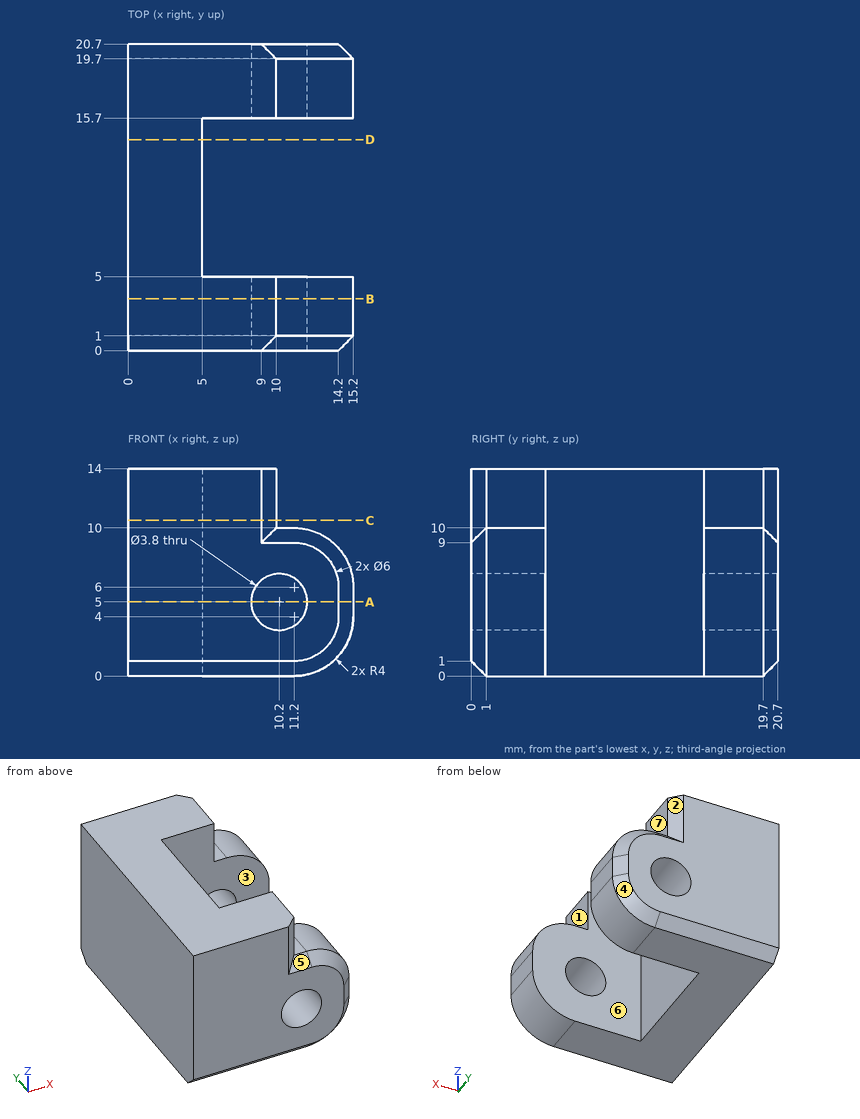
Geometry: see drawing. Coordinates: mm, zero at the bounding-box minimum. A direction names the side the tool comes from. Coordinates: 2 decimals unless noted, no trailing zeros. Loops run counter-clockwise (first coordinate to the right, second up) from the corner with the lowest first, then second, coordinate; pieces in that order, holes last. Notation, with made-up numbers: M 6.25,28 L 58.25,28 A25 cw 58.25,51 Z; hole C 57.25,5.25 d4. An arc over 180 degrees is marked long. Answer in a Markdown table with one row per item.
Q1. Draft query along Y for the marked faces 4, 5, 6 and 7. Return one class per face: pulls with the +Y half, pulls with the -Y half, needs draft (parallel to the pull), parting line crosses it, or undercut.
Answers below:
| item | result |
|---|---|
| face 4 | pulls with the +Y half |
| face 5 | pulls with the -Y half |
| face 6 | undercut |
| face 7 | needs draft |
Q2. Set-up query: the marked faces 1, 2 and 3. Return all of +Z, -Z, +X, -X, +Y, -Y with unobstructed straight access to the full face (end or side cutting, diameter ignored); none if empty.
Answers below:
| item | result |
|---|---|
| face 1 | +Z, +X, +Y, -Y |
| face 2 | +Z, +X, +Y |
| face 3 | +Z, -Z, +X |
Q3. Ray query, probe 1 along Z at (x, y) = (10.2, 3.65); probe 2 along Y at (x, z) = (6, 13); probe 3 along X at (y, z) = (14, 6.5). Return the intervals inside material, ascending. Write a range as from..to.
Answers below:
| item | result |
|---|---|
| probe 1 | z = 0..3.1, 6.9..10 |
| probe 2 | y = 0..5, 15.7..20.7 |
| probe 3 | x = 0..5 |
Q4. Section B-B on y = 3.5. Return the cut outline in (x, z), plus the area to 3 significant figures.
Answers below:
| item | result |
|---|---|
| outline | M 0,0 L 11.2,0 A4 ccw 15.2,4 L 15.2,6 A4 ccw 11.2,10 L 10,10 L 10,14 L 0,14 Z; hole C 10.2,5 d3.8 |
| area | 174 mm^2 |
Q5. Section A-A on z = 5. Return the cut outline in (x, y).
Answers below:
| item | result |
|---|---|
| outline | M 0,0 L 8.3,0 L 8.3,5 L 5,5 L 5,15.7 L 8.3,15.7 L 8.3,20.7 L 0,20.7 Z; M 12.1,0 L 14.2,0 L 15.2,1 L 15.2,5 L 12.1,5 Z; M 12.1,15.7 L 15.2,15.7 L 15.2,19.7 L 14.2,20.7 L 12.1,20.7 Z |
Q6. First-contact query: pin 1 (3 mm diameter, centred on x = 9.5, z = 9.5, fed in from -Y); pin 2 (5 mm diameter, centred on x = 12, y = 13.5, fed in from +Z); pin 3 (1.2 mm diameter, centred on y = 18.5, z = 12, fed in from +X); pin 4 (5 mm diameter, centred on x = 8, y = 12, fed in from +Z). Flat tips, straight axial feed; report the tip coordinate or a pass-through.
Answers below:
| item | result |
|---|---|
| pin 1 | stops at y = 0 |
| pin 2 | stops at z = 10 |
| pin 3 | stops at x = 10 |
| pin 4 | passes through |
Q7. Section D-D on y = 14.25. Return the cut outline in (x, z).
Answers below:
| item | result |
|---|---|
| outline | M 0,0 L 5,0 L 5,14 L 0,14 Z |
Q8. Section C-C on z = 10.5. Return the cut outline in (x, y), plus the area to 4 significant figures.
Answers below:
| item | result |
|---|---|
| outline | M 0,0 L 9,0 L 10,1 L 10,5 L 5,5 L 5,15.7 L 10,15.7 L 10,19.7 L 9,20.7 L 0,20.7 Z |
| area | 152.5 mm^2 |
